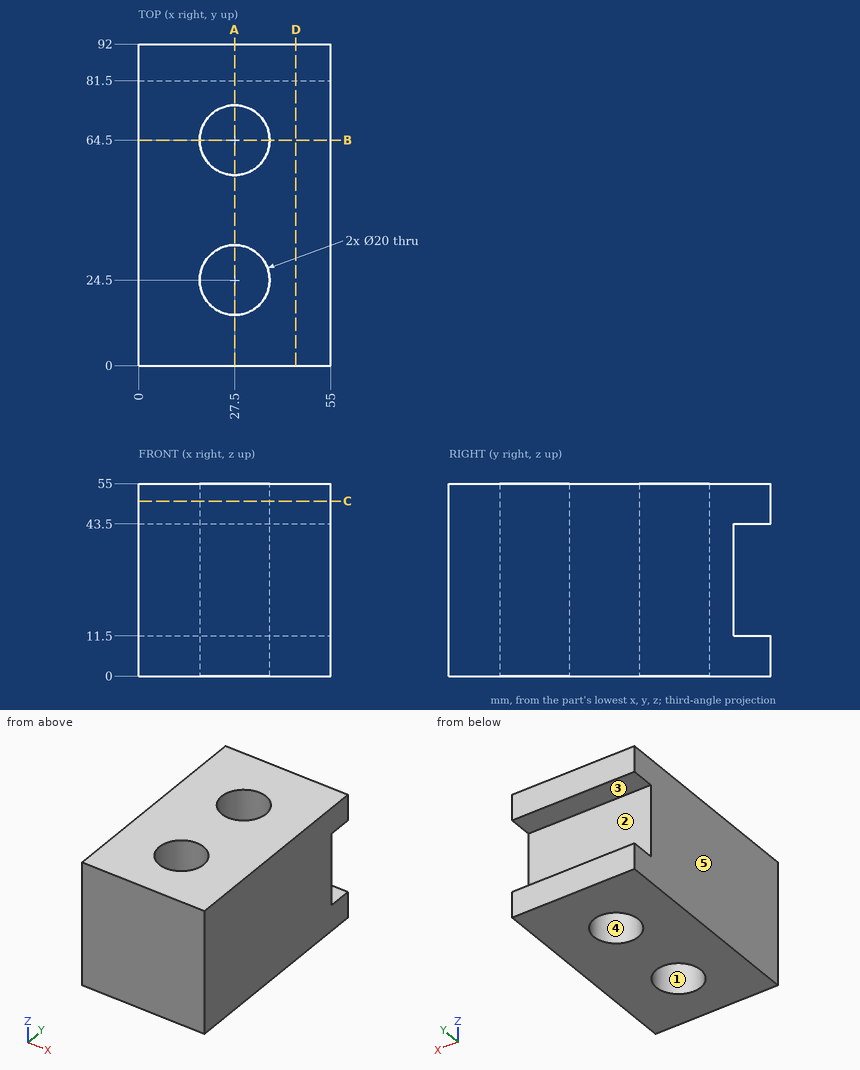
Drawing for the job (mm, zero at the part's lowest x, y, z). A direction names the side the tool comes from. Coordinates: 2 decimals unless noted, no trailing zeros. Loops run counter-clockwise (first coordinate to the right, second up) from the corner with the lowest first, then second, coordinate; pieces in that order, holes last. Notation, with made-up numbers: (79, 40.25) - (87, 40.25) arc R13 ccw to (87, 46.25) - close; hole circle Ø9 at (-35, 12.25). An arc over 180 degrees is marked (long way). Return JSON: item names as keys, results as strings.
1. 3-axis set-ups, long thin cutter, end or side, ignore diameter. For the marked faces 1 and 2: which of +Z, -Z, +X, -X, +Y, -Y reach the whole face in a straight line?
Result:
{"face 1": "+Z, -Z", "face 2": "+X, -X, +Y"}
2. Probe L1, parallel to Y at x = 27, z = 38; L2, parallel to X at y = 24.5, z = 42; L3, parallel to Y at x = 36.5, z = 48.5. List the from-to ranges inside material, lowest first. Write a range as from..to.
Result:
{"L1": "y = 0..14.51, 34.49..54.51, 74.49..81.5", "L2": "x = 0..17.5, 37.5..55", "L3": "y = 0..20.14, 28.86..60.14, 68.86..92"}
3. Drop flat-ended pins along their axis: pin 1 (2 mm diameter, centred on x = 8, z = 9.5, fed in from -Y); pin 2 (9.5 mm diameter, centred on x = 14.5, z = 27, fed in from +Y). Give the stop position or say it passes through.
Result:
{"pin 1": "stops at y = 0", "pin 2": "stops at y = 81.5"}
4. Band-saw the part on B-B (y = 64.5). Give the cut face in (x, z), and give its area (4 significant figures).
Result:
{"outline": "(0, 0) - (17.5, 0) - (17.5, 55) - (0, 55) - close; (37.5, 0) - (55, 0) - (55, 55) - (37.5, 55) - close", "area": "1,925 mm2"}
5. Mould opens along X. For the marked faces 3, 4 and 5 say: released by +X, released by -X, zero draft, split by the parting line, or undercut.
Result:
{"face 3": "zero draft", "face 4": "undercut", "face 5": "released by -X"}
6. Band-saw the part on C-C (z = 50). Give the cut face in (x, y), and give its area (3 significant figures).
Result:
{"outline": "(0, 0) - (55, 0) - (55, 92) - (0, 92) - close; hole circle Ø20 at (27.5, 24.5); hole circle Ø20 at (27.5, 64.5)", "area": "4,430 mm2"}
7. Band-saw the part on D-D (x = 45). Give the cut face in (y, z), and give its area (3 significant figures).
Result:
{"outline": "(0, 0) - (92, 0) - (92, 11.5) - (81.5, 11.5) - (81.5, 43.5) - (92, 43.5) - (92, 55) - (0, 55) - close", "area": "4,720 mm2"}
8. Band-saw the part on A-A (x = 27.5). Give the cut face in (y, z), and give its area (3 significant figures).
Result:
{"outline": "(0, 0) - (14.5, 0) - (14.5, 55) - (0, 55) - close; (34.5, 0) - (54.5, 0) - (54.5, 55) - (34.5, 55) - close; (74.5, 0) - (92, 0) - (92, 11.5) - (81.5, 11.5) - (81.5, 43.5) - (92, 43.5) - (92, 55) - (74.5, 55) - close", "area": "2,520 mm2"}
